from build123d import *

# Parameters (mm, degrees)
EXTRUDE_1_DEPTH     = 5
CUT_EXTRUDE_1_DEPTH = 3
CUT_EXTRUDE_2_DEPTH = 6.5


with BuildPart() as part:
    # Эскиз1 → Бобышка-Вытянуть1 (new body, symmetric)
    with BuildSketch(Plane.XY):
        Polygon((5, 0), (-5, 0), (-5, -3), (-9.75, -3), (-9.75, -8.5), (9.75, -8.5), (9.75, -3), (5, -3), align=None)
    extrude(amount=EXTRUDE_1_DEPTH, both=True)

    # Эскиз3 → Отверстие обработанное метчиком M51 (revolve, cut)
    with BuildSketch(Plane(origin=(0, 0, 0), x_dir=(0, 0, 1), z_dir=(1, 0, 0))):
        Polygon((0, 0), (0, 8.5), (3.1, 8.5), (2.1, 7.5), (2.1, 1), (3.1, 0), align=None)
    revolve(axis=Axis((0, 6.35, 0), (0, -1, 0)), mode=Mode.SUBTRACT)

    # Эскиз4 → Вырез-Вытянуть1 (cut)
    with BuildSketch(Plane(origin=(0, 0, 0), x_dir=(1, 0, 0), z_dir=(0, 1, 0))):
        with BuildLine():
            Line((-5, 5), (-5, 0))
            ThreePointArc((-5, 0), (-3.535533906, 3.535533906), (0, 5))
            Line((0, 5), (-5, 5))
        make_face()
        with BuildLine():
            Line((0, -5), (5, -5))
            Line((5, -5), (5, 0))
            ThreePointArc((5, 0), (3.535533906, -3.535533906), (0, -5))
        make_face()
    extrude(amount=-CUT_EXTRUDE_1_DEPTH, mode=Mode.SUBTRACT)

    # Эскиз5 → Вырез-Вытянуть2 (cut, through all)
    with BuildSketch(Plane(origin=(0, -3, 0), x_dir=(1, 0, 0), z_dir=(0, 1, 0))):
        with BuildLine():
            Line((-9.75, 0), (-9.75, 5))
            Line((-9.75, 5), (-8.370334521, 5))
            ThreePointArc((-8.370334521, 5), (-9.398756875, 2.59342808), (-9.75, 0))
        make_face()
        with BuildLine():
            Line((9.75, 0), (9.75, -5))
            Line((9.75, -5), (8.370334521, -5))
            ThreePointArc((8.370334521, -5), (9.398756875, -2.59342808), (9.75, 0))
        make_face()
    extrude(amount=-CUT_EXTRUDE_2_DEPTH, mode=Mode.SUBTRACT)

    # Вырез-По траектории1: sweep along a path in Эскиз7
    with BuildLine(Plane.XZ.offset(8.5)) as sweep_1_path:
        Line((0, 9.75), (-9.75, 9.75))
        Line((-9.75, 9.75), (-9.75, 0))
        ThreePointArc((-9.75, 0), (-6.894291117, -6.894291117), (0, -9.75))
        Line((0, -9.75), (9.75, -9.75))
        Line((9.75, -9.75), (9.75, 0))
        ThreePointArc((9.75, 0), (6.894291117, 6.894291117), (0, 9.75))
    # Эскиз6 → Вырез-По траектории1 (sweep, cut)
    with BuildSketch(Plane.XY.offset(5)):
        Polygon((-9.75, -5.5), (-9.75, -8.5), (-5, -8.5), align=None)
    sweep(path=sweep_1_path.line, transition=Transition.RIGHT, mode=Mode.SUBTRACT)


solid = part.part
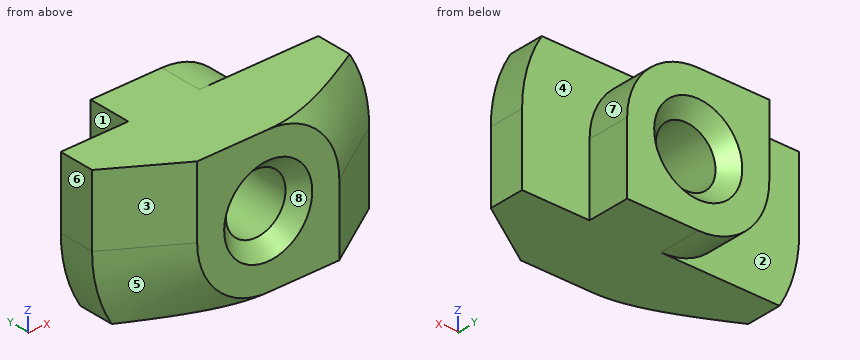
Can you work these out from the model? Positions are in its coordinate system, mm. Face numbers are marked on the shaded views. A direction names the side the tool comes from. Round coordinates to 2 decimals unless told otherwise and drop trailing zeros. Loops run counter-clockwise (first coordinate to the right, second up) from the corner with the lowest first, then second, coordinate; pieces in that order, holes last. Notation, with made-up numbers: (55, -29.5) - (90, -29.5) arc R25 cw to (90, -13.5) - close; hole circle Ø5 at (10, 31.25). An arc over 180 degrees is marked (long way). Answer in a Markdown table with one row per item. Add a question column.
Q1. We'd pull the mould along Z, two halves only. Please class the marked faces 5, 6, 7 and 8: pulls with the +Z half, pulls with the -Z half, needs draft (parallel to the pull), parting line crosses it, or undercut.
Q2. I need wall thicknesses on L1, parallel to Z at x = 0, y = -5.5; L2, parallel to X at y = -1.25, z = -1; L3, parallel to X at y = -6, z = 0. Which ranges of each line are inside material? Lowest first, please.
Q3. I want a section at B-B on y = -5.75. List the corners of the cut face in (x, z) for me, and give its area (3 significant figures).
Q4. For pin 1 Ø3.5 at (y, z) = (-1, 1.5) entering from -X; pin 2 Ø1 at (x, z) = (2, -0.5) entering from -Y; pin 3 Ø5.5 at (x, z) = (0, 0) entering from -Y, each with a flat end and sliding along its axis, tell me the tip position at first contact or that it passes through.
Q5. Which directions (+Z, -Z, +X, -X, +Y, -Y) give clear straight access to the entire face, cutting with the end or side of a thin tool? Please do the marked faces 1, 2, 3 and 4.
Q6. I want a section at A-A on y = -4.5. List the corners of the cut face in (x, z) for me.
A:
| question | item | result |
|---|---|---|
| 1 | face 5 | pulls with the -Z half |
| 1 | face 6 | needs draft |
| 1 | face 7 | pulls with the +Z half |
| 1 | face 8 | undercut |
| 2 | L1 | -5 to -2.1, 2.1 to 5 |
| 2 | L2 | -4.9 to -1.85, 1.85 to 5 |
| 2 | L3 | -8.96 to -2.1, 2.1 to 8.96 |
| 3 | outline | (-9.35, 0) arc R9.35 ccw to (-7.91, -5) - (9.35, -5) - (9.35, 0) arc R9.35 ccw to (7.91, 5) - (-9.35, 5) - close; hole circle Ø4.2 at (0, 0) |
| 3 | area | 169 mm^2 |
| 4 | pin 1 | x = -5 |
| 4 | pin 2 | y = -7.96 |
| 4 | pin 3 | y = -8.15 |
| 5 | face 1 | +Z, -Z, -X, +Y |
| 5 | face 2 | -Z, -X, +Y |
| 5 | face 3 | +Z, -Z, -X, -Y |
| 5 | face 4 | +Z, +X, +Y |
| 6 | outline | (-9.75, 0) arc R9.75 ccw to (-8.37, -5) - (9.75, -5) - (9.75, 0) arc R9.75 ccw to (8.37, 5) - (-9.75, 5) - close; hole circle Ø4.2 at (0, 0) |
